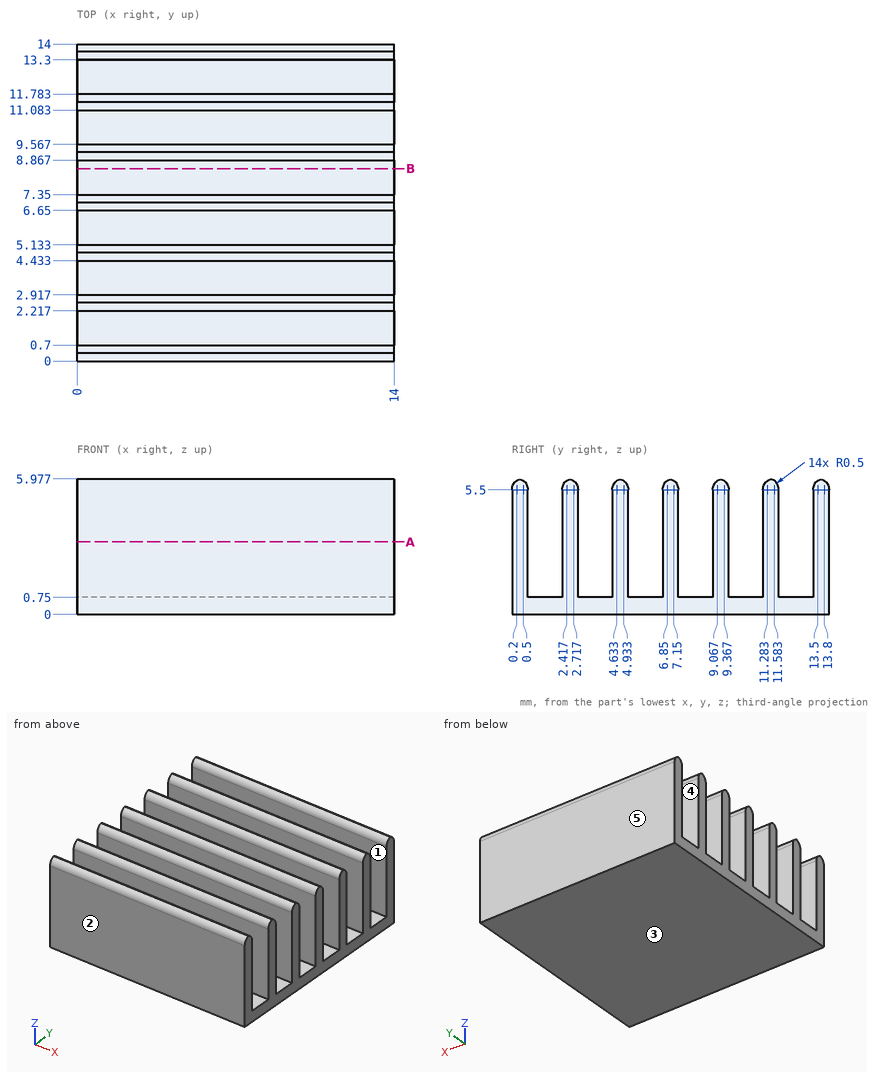
Geometry check sheet. Reference: drawing and pictorial views, mm from the part's lowest x, y, z. A direction names the side the tool comes from. Round coordinates to 2 decimals unless told otherwise and drop trailing zeros. Loops run counter-clockwise (first coordinate to the right, second up) from the corner with the lowest first, then second, coordinate; pieces in that order, holes last.
1. Sectioned sample at A-A on z = 3.2. Record the boundary of the cut face in (x, y).
2. Scan lines: probe 1 along Z at (x, y) = (9.25, 12.5); probe 2 along Z at (x, y) = (9.5, 9.25) (1 decimal). Record each from-to range of solid material in increasing order.
3. Set-up check for the marked faces 4 and 5: record each of +Z, -Z, +X, -X, +Y, -Y from which the full face is reachable in a straight line by a thin tool's end or side.
4. Sectioned sample at B-B on y = 8.5. Record the boundary of the cut face in (x, z), and give its area (3 significant figures).
5. Mould release check, pull along Y, two halves, no side actions. Record for the marked faces 1, 2 and 3: released by +Y, released by -Y, zero draft, split by the parting line, or undercut.
6. Gauge pin test, flat ends, axial feed: pin 1 Ø0.8 at (x, y) = (6.5, 4) entering from +Z; pin 2 Ø1 at (x, z) = (7, 1) entering from -Y. Record the tip position at first contact, or that the pin passes through.
Recorded:
1. outline: (0, 0) - (14, 0) - (14, 0.7) - (0, 0.7) - close; (0, 2.22) - (14, 2.22) - (14, 2.92) - (0, 2.92) - close; (0, 4.43) - (14, 4.43) - (14, 5.13) - (0, 5.13) - close; (0, 6.65) - (14, 6.65) - (14, 7.35) - (0, 7.35) - close; (0, 8.87) - (14, 8.87) - (14, 9.57) - (0, 9.57) - close; (0, 11.08) - (14, 11.08) - (14, 11.78) - (0, 11.78) - close; (0, 13.3) - (14, 13.3) - (14, 14) - (0, 14) - close
2. probe 1: z = 0 to 0.75
2. probe 2: z = 0 to 6
3. face 4: +Z, +X, -X
3. face 5: +Z, -Z, +X, -X, +Y
4. outline: (0, 0) - (14, 0) - (14, 0.75) - (0, 0.75) - close
4. area: 10.5 mm2
5. face 1: undercut
5. face 2: released by -Y
5. face 3: zero draft
6. pin 1: stops at z = 0.75
6. pin 2: stops at y = 0
